Geometry check sheet. Reference: the model listing, model coordinates, mm. A direction names the side the tool comes from. Round coordinates to 2 decimals unless told otherwise and drop trailing zeros. Order: outer loops, then holes, each group sorted by start corner. A loop starts at its lowest first (then second) coordinate and runs counter-clockwise, first axis right, second up.
(1) Gauge pin test, flat ends, axial feed: P1, Ø12, axis at x = 10, y = 43, coming from the +Z side; P2, Ø5, axis at y = 8.5, z = 16.5, coming from the +X side; P3, Ø1.5, axis at x = 60.5, y = 40, coming from the -Z side. Record the tip position at first contact, or that the pin passes through.
(2) Cross-section at A-A on y = 22. Enter the section's corners in (x, z).
(3) Cross-section at D-D on y = 2.5. Enter the section's corners in (x, z), and give its area (3 significant figures).
(4) Set-up check for faces 1 (the face through (72, 23, 6)), 2 (the face through (61, 23, 0)), 3 (the face through (39, 46, 6)): record each of +Z, -Z, +X, -X, +Y, -Y from which the full face is reachable in a straight line by a thin tool's end or side.
(5) Draft check along Y on faces 4 (the face through (48, 23, 12)), 5 (the face through (31.7, 48, 40.7)), 6 (the face through (13, 38, 6)), 7 (the face through (40, 5, 20)). Enter one of: pulls with the +Y half, pulls with the -Y half, needs draft (parallel to the pull), parting line crosses it, or undercut.
(6) Cross-section at B-B on x = 67. Enter the section's corners in (y, z), and give its area (3 significant figures).
(7) Cross-section at C-C on z = 5. Enter the section's corners in (x, y).
(8) Thickness scan on L1, parallel to Z at x = 40, y = 14; L2, parallel to Z at x = 8, y = 2; L3, parallel to X at y = 19, z = 16. Record the ranges inside material, lowest first.
from build123d import *

# Parameters (mm, degrees)
F0_W      = 80
F0_H      = 46
F1_DEPTH  = 12
F3_DEPTH  = 3
F5_DEPTH  = 12
F6_W      = 36
F6_H      = 46
F6_H_2    = 2
F7_DEPTH  = 51
F8_R      = 9
F9_DEPTH  = 51
F11_DEPTH = 7
F13_DEPTH = 7


with BuildPart() as f1:
    # F0 (on Top) → F1 (new body)
    with BuildSketch(Plane.XY):
        with Locations((40, 23)):
            Rectangle(F0_W, F0_H)
    extrude(amount=F1_DEPTH)

    # F2 (on face) → F3 (join)
    with BuildSketch(Plane(origin=(0, 0, 0), x_dir=(1, 0, 0), z_dir=(0, 0, -1))):
        Polygon((30, -46), (40, -46), (50, -46), (50, 0), (30, 0), align=None)
    extrude(amount=F3_DEPTH)

    # F4 (on face) → F5 (cut)
    with BuildSketch(Plane.XY.offset(12)):
        with BuildLine():
            Line((8, 33), (8, 13))
            ThreePointArc((8, 13), (13, 8), (18, 13))
            Line((18, 13), (18, 33))
            ThreePointArc((18, 33), (13, 38), (8, 33))
        make_face()
        with BuildLine():
            ThreePointArc((72, 33), (67, 38), (62, 33))
            Line((62, 33), (62, 13))
            ThreePointArc((62, 13), (67, 8), (72, 13))
            Line((72, 13), (72, 33))
        make_face()
    extrude(amount=-F5_DEPTH, mode=Mode.SUBTRACT)

    # F6 (on face) → F7 (join)
    with BuildSketch(Plane.XY.offset(12)):
        with Locations((40, 23)):
            Rectangle(F6_W, F6_H)
        with Locations((40, -1)):
            Rectangle(F6_W, F6_H_2)
        with Locations((40, 47)):
            Rectangle(F6_W, F6_H_2)
    extrude(amount=F7_DEPTH)

    # F8 (on face) → F9 (cut)
    with BuildSketch(Plane.XZ.offset(2)):
        with BuildLine():
            Line((22, 63), (22, 45))
            ThreePointArc((22, 45), (27.2720779386, 57.7279220614), (40, 63))
            Line((40, 63), (22, 63))
        make_face()
        with BuildLine():
            ThreePointArc((40, 63), (52.7279220614, 57.7279220614), (58, 45))
            Line((58, 45), (58, 63))
            Line((58, 63), (40, 63))
        make_face()
        with BuildLine():
            ThreePointArc((58, 45), (54.6969384567, 34.6076951546), (46, 28.0294372515))
            Line((46, 28.0294372515), (46, 12))
            Line((46, 12), (58, 12))
            Line((58, 12), (58, 45))
        make_face()
        with BuildLine():
            Line((34, 12), (34, 28.0294372515))
            ThreePointArc((34, 28.0294372515), (25.3030615433, 34.6076951546), (22, 45))
            Line((22, 45), (22, 12))
            Line((22, 12), (34, 12))
        make_face()
        with Locations((40, 45)):
            Circle(F8_R)
    extrude(amount=-F9_DEPTH, mode=Mode.SUBTRACT)

    # F10 (on face) → F11 (cut)
    with BuildSketch(Plane.XZ.offset(2)):
        with BuildLine():
            Line((34, 12), (46, 12))
            Line((46, 12), (46, 28.0294372515))
            ThreePointArc((46, 28.0294372515), (40, 27), (34, 28.0294372515))
            Line((34, 28.0294372515), (34, 12))
        make_face()
    extrude(amount=-F11_DEPTH, mode=Mode.SUBTRACT)

    # F12 (on face) → F13 (cut)
    with BuildSketch(Plane(origin=(0, 48, 0), x_dir=(-1, 0, 0), z_dir=(0, 1, 0))):
        with BuildLine():
            Line((-46, 28.0294372515), (-46, 12))
            Line((-46, 12), (-34, 12))
            Line((-34, 12), (-34, 28.0294372515))
            ThreePointArc((-34, 28.0294372515), (-40, 27), (-46, 28.0294372515))
        make_face()
    extrude(amount=-F13_DEPTH, mode=Mode.SUBTRACT)


solid = f1.part
Found:
1. P1: stops at z = 12
1. P2: stops at x = 46
1. P3: stops at z = 0
2. outline: (0, 0) - (8, 0) - (8, 12) - (0, 12) - close; (18, 0) - (30, 0) - (30, -3) - (50, -3) - (50, 0) - (62, 0) - (62, 12) - (46, 12) - (46, 28.03) arc R18 ccw (long way) to (34, 28.03) - (34, 12) - (18, 12) - close; (72, 0) - (80, 0) - (80, 12) - (72, 12) - close; hole circle Ø18 at (40, 45)
3. outline: (0, 0) - (30, 0) - (30, -3) - (50, -3) - (50, 0) - (80, 0) - (80, 12) - (0, 12) - close; circle Ø36 at (40, 45); hole circle Ø18 at (40, 45)
3. area: 1,780 mm2
4. face 1: +Z, -Z
4. face 2: -Z, +X, +Y, -Y
4. face 3: -Z, +X, -X, +Y
5. face 4: needs draft
5. face 5: pulls with the +Y half
5. face 6: undercut
5. face 7: pulls with the -Y half
6. outline: (0, 0) - (8, 0) - (8, 12) - (0, 12) - close; (38, 0) - (46, 0) - (46, 12) - (38, 12) - close
6. area: 192 mm2
7. outline: (0, 0) - (80, 0) - (80, 46) - (0, 46) - close; hole (8, 13) arc R5 ccw to (18, 13) - (18, 33) arc R5 ccw to (8, 33) - close; hole (62, 13) arc R5 ccw to (72, 13) - (72, 33) arc R5 ccw to (62, 33) - close
8. L1: z = -3 to 36, 54 to 63
8. L2: z = 0 to 12
8. L3: x = 34 to 46
